from build123d import *

# Parameters (mm, degrees)
CROQUIS1_W              = 35
CROQUIS1_H              = 35
CROQUIS1_R              = 1.25
CROQUIS1_R_2            = 6.5
SALIENTE_EXTRUIR1_DEPTH = 5
CORTAR_EXTRUIR1_DEPTH   = 2


with BuildPart() as part:
    # Croquis1 → Saliente-Extruir1 (new body)
    with BuildSketch(Plane.XY):
        Rectangle(CROQUIS1_W, CROQUIS1_H)
        with Locations((-15.37, 15.37)):
            Circle(CROQUIS1_R, mode=Mode.SUBTRACT)
        with Locations((15.37, 15.37)):
            Circle(CROQUIS1_R, mode=Mode.SUBTRACT)
        with Locations((15.37, -15.37)):
            Circle(CROQUIS1_R, mode=Mode.SUBTRACT)
        with Locations((-15.37, -15.37)):
            Circle(CROQUIS1_R, mode=Mode.SUBTRACT)
        Circle(CROQUIS1_R_2, mode=Mode.SUBTRACT)
        with Locations((13.3, 0)):
            Circle(CROQUIS1_R, mode=Mode.SUBTRACT)
        with Locations((-13.3, 0)):
            Circle(CROQUIS1_R, mode=Mode.SUBTRACT)
    extrude(amount=SALIENTE_EXTRUIR1_DEPTH)

    # Croquis2 → Cortar-Extruir1 (cut)
    with BuildSketch(Plane.XY.offset(5)):
        Polygon((-13.3, 3.464101615), (-16.3, 1.732050808), (-16.3, -1.732050808), (-13.3, -3.464101615), (-10.3, -1.732050808), (-10.3, 1.732050808), align=None)
        Polygon((13.3, 3.464101615), (10.3, 1.732050808), (10.3, -1.732050808), (13.3, -3.464101615), (16.3, -1.732050808), (16.3, 1.732050808), align=None)
    extrude(amount=-CORTAR_EXTRUIR1_DEPTH, mode=Mode.SUBTRACT)


solid = part.part
Design review of the part built by this model. Coordinates are the model's own, in mm. A direction names the side the tool comes from. Give positions to 0.01 mm unless a question says otherwise; leave off trailing zeros. Loops run counter-clockwise (first coordinate to the right, second up) from the corner with the lowest first, then second, coordinate; pieces in that order, holes last. Notation, with made-up numbers: M -39,54 L -34,54 A32 cw -34,81 Z; hole C 36,-3 d4. An arc over 180 degrees is marked long. Write item = value, one per line.
Q1. To check wall thickness, follow line 1 (Y direction, x = 15.37, z = 1.55); line 2 (Y direction, x = -15, z = 3.8); line 3 (Y direction, x = -13.3, z = 2.05). State the ranges of each line that lie inside material, in increasing order. Write a range as [from, to].
Output values:
line_1 = [-17.5, -16.62], [-14.12, 14.12], [16.62, 17.5]
line_2 = [-17.5, -16.56], [-14.18, -2.48], [2.48, 14.18], [16.56, 17.5]
line_3 = [-17.5, -1.25], [1.25, 17.5]
Q2. We need section D-D (x = -15). Give the boundary of the cut face in (y, z).
Output values:
outline = M -17.5,0 L -16.56,0 L -16.56,5 L -17.5,5 Z; M -14.18,0 L 14.18,0 L 14.18,5 L 2.48,5 L 2.48,3 L -2.48,3 L -2.48,5 L -14.18,5 Z; M 16.56,0 L 17.5,0 L 17.5,5 L 16.56,5 Z
Q3. Draft analysis for pull direction X (two halves, no side actions). For faces 3 (the flat face through (14.8, 2.6, 4)), 4 (the flat face through (-17.5, 0, 2)), 5 (the flat face through (8, 0, 5)), 6 (the flat face through (-14.8, 2.6, 4)), state which applies: +X half, -X half, draft (parallel to the pull), parting line (faces both ways), or undercut.
Output values:
face_3 = undercut
face_4 = -X half
face_5 = draft
face_6 = undercut
Q4. We need section A-A (x = 0). Give the boundary of the cut face in (y, z), plus the area to 3 significant figures.
Output values:
outline = M -17.5,0 L -6.5,0 L -6.5,5 L -17.5,5 Z; M 6.5,0 L 17.5,0 L 17.5,5 L 6.5,5 Z
area = 110 mm^2
Q5. We need section B-B (z = 4.15). Give the boundary of the cut face in (x, y), plus the area to 3 significant figures.
Output values:
outline = M -17.5,-17.5 L 17.5,-17.5 L 17.5,17.5 L -17.5,17.5 Z; hole C -15.37,-15.37 d2.5; hole C -15.37,15.37 d2.5; hole M -16.3,-1.73 L -13.3,-3.46 L -10.3,-1.73 L -10.3,1.73 L -13.3,3.46 L -16.3,1.73 Z; hole C 0,0 d13; hole M 10.3,-1.73 L 13.3,-3.46 L 16.3,-1.73 L 16.3,1.73 L 13.3,3.46 L 10.3,1.73 Z; hole C 15.37,-15.37 d2.5; hole C 15.37,15.37 d2.5
area = 1,010 mm^2
Q6. Insertion check: pin 1 (3 mm diameter, centred on x = -13.3, y = 0, fed in from +Z); pin 2 (1.5 mm diameter, centred on x = 13.3, y = 0, fed in from +Z). Each pin has a flat end and moves straight along its axis. Give the tip position at first contact, or say it passes through.
Output values:
pin_1 = 3
pin_2 = through
Q7. For faces 1 (the cylindrical face through (-14.18, 15.75, 2.46)), 2 (the flat face through (-14.8, -2.6, 4)), list the 3-axis set-ups (+Z, -Z, +X, -X, +Y, -Y) from which the entire face can be reached by the end or side of a thin tool; tool diameter is ignored.
Output values:
face_1 = +Z, -Z
face_2 = +Z
Q8. We need section C-C (y = 4.5). Give the boundary of the cut face in (x, z).
Output values:
outline = M -17.5,0 L -4.69,0 L -4.69,5 L -17.5,5 Z; M 4.69,0 L 17.5,0 L 17.5,5 L 4.69,5 Z
